Autodesk Inventor part; units mm, degrees
ref_plane "YZ Plane" through (0, 0, 0) normal (1, 0, 0) x (0, 1, 0)
ref_plane "XZ Plane" through (0, 0, 0) normal (0, 1, 0) x (-1, 0, 0)
ref_plane "XY Plane" through (0, 0, 0) normal (0, 0, 1) x (1, 0, 0)
sketch "Sketch3" plane through (0, 0, 0) normal (0, 0, 1) x (1, 0, 0)
  circle A0 centre (0, 0) radius 9.525
  dimension "d7" = 19.05
extrude "Extrusion3" add sketch "Sketch3" along normal blind 38.1
sketch "Sketch4" plane through (0, 0, 38.1) normal (0, 0, 1) x (1, 0, 0)
  line L0 (5.2594, 3.6744) -> (5.8118, -2.7176)
  line L1 (5.8118, -2.7176) -> (0.5524, -6.392)
  line L2 (0.5524, -6.392) -> (-5.2594, -3.6744)
  line L3 (-5.2594, -3.6744) -> (-5.8118, 2.7176)
  line L4 (-5.8118, 2.7176) -> (-0.5524, 6.392)
  line L5 (-0.5524, 6.392) -> (5.2594, 3.6744)
  point P0 (0, 0)
  point P1 (0, 0)
  dimension "d10" = 11.1125
extrude "Extrusion4" cut sketch "Sketch4" against normal blind 5.715
sketch "Sketch5" plane through (0, 0, 32.385) normal (0, 0, 1) x (1, 0, 0)
  circle A0 centre (0, 0) radius 2.3749
  dimension "d13" = 4.7498
hole "Hole1" at (0, 0, 32.385) direction (0, 0, -1) diameter 4.7498 depth 13.335 tip angle 118
sketch "Sketch6" plane through (0, 0, 0) normal (0, 0, -1) x (-1, 0, 0)
  point P0 (0, 0)
sketch "Sketch7" plane through (0, 0, 0) normal (0, 0, -1) x (-1, 0, 0)
  point P0 (0, 0)
sketch "Sketch8" plane through (0, 0, 0) normal (0, 0, -1) x (-1, 0, 0)
  arc A0 (-1.6801, 1.905) -> (1.6801, 1.905) centre (0, 0) ccw
  line L0 (-1.6801, 1.905) -> (1.6801, 1.905)
  dimension "d21" = 5.08
extrude "Extrusion5" cut sketch "Sketch8" against normal blind 19.05
properties part number "Vertical Sedder motor and rail coupler"
Design review of the part built by this model. Coordinates are the model's own, in mm. A direction names the side the tool comes from. Coordinates: 2 decimals unless noted, no trailing zeros. Order: outer loops, then holes, each group sorted by start corner. A loop starts at its lowest first (then second) coordinate and runs counter-clockwise, first axis right, second up. Notation, with made-up numbers: M 24.25,-38 L 83.25,-38 A10 ccw 83.25,-21 Z; hole C 50.25,86.5 d8. An arc over 180 degrees is marked long. Answer as a JSON object with one key per item and string values. Group by question number.
1) Add section A-A, the plane z = 34. Write out the cut boundary in (x, y) (3 decimals), then the cut area to 3 significant figures.
2) Wall thickness on L1, parallel to Y at x = 0, z = 14.25 (3 decimals); L2, parallel to Y at x = 0, z = 22.5 (3 decimals); L3, parallel to Z at x = -2.75, y = -3.5 (3 decimals): over which ranges is each line inside the solid? List them lowest first.
3) Add section D-D, the plane x = 3.5. Write out the cut boundary in (y, z) (3 decimals).
4) For pin 1 (8 mm diameter, centred on y = 7, z = 25, fed in from +X); pin 2 (6 mm diameter, centred on x = -4, z = 9.5, fed in from +Y); pin 3 (1.5 mm diameter, centred on y = -6, z = 12, fed in from -X), all flat-tipped, find the tip position at first contact; note any pin that passes through.
5) Add section B-B, the plane y = -1. Write out the cut boundary in (x, z) (3 decimals), then the cut area to 3 significant figures.
6) Mouldability with a two-part tool opening along X and no side actions: class faces 4 (the cylindrical face through (-7.559, 5.796, 18.783)), 5 (the flat face through (4.1, -4.1, 38.1)), 6 (the flat face through (-5.53, -0.52, 35.28)) as pulls with the +X half, pulls with the -X half, needs draft (parallel to the pull), parting line crosses it, or undercut.
7) Add section C-C, the plane x = 0. Write out the cut boundary in (y, z) (3 decimals), then the cut area to 3 significant figures.
8) Tool access review of faces 1 (the flat face through (-0.1, 2.3, 0)), 2 (the flat face through (0, 1.905, 9)), 3 (the flat face through (-2.313, -5.052, 35.283)): name each direction out of +Z, -Z, +X, -X, +Y, -Y from which nothing blocks a thin tool from reaching the whole face with its end or side.
Computed values:
{
 "1": {"outline": "C 0,0 d19.05; hole M -5.812,2.718 L -5.259,-3.674 L 0.552,-6.392 L 5.812,-2.718 L 5.259,3.674 L -0.552,6.392 Z", "area": "178 mm^2"},
 "2": {"L1": "y = -9.525 to -2.54, 1.905 to 9.525", "L2": "y = -9.525 to -2.375, 2.375 to 9.525", "L3": "z = 0 to 32.385"},
 "3": {"outline": "M -8.859,0 L 8.859,0 L 8.859,38.1 L 4.497,38.1 L 4.497,32.385 L -4.333,32.385 L -4.333,38.1 L -8.859,38.1 Z"},
 "4": {"pin 1": "stops at x = 9.04", "pin 2": "stops at y = 9.47", "pin 3": "stops at x = -7.95"},
 "5": {"outline": "M -9.472,0 L -2.335,0 L -2.335,19.05 L -2.154,19.05 L -2.154,32.385 L -5.491,32.385 L -5.491,38.1 L -9.472,38.1 Z; M 2.154,19.05 L 2.335,19.05 L 2.335,0 L 9.472,0 L 9.472,38.1 L 5.663,38.1 L 5.663,32.385 L 2.154,32.385 Z", "area": "512 mm^2"},
 "6": {"face 4": "parting line crosses it", "face 5": "needs draft", "face 6": "undercut"},
 "7": {"outline": "M -9.525,0 L -2.54,0 L -2.54,19.05 L -2.375,19.05 L -2.375,32.385 L -6.134,32.385 L -6.134,38.1 L -9.525,38.1 Z; M 1.905,0 L 9.525,0 L 9.525,38.1 L 6.134,38.1 L 6.134,32.385 L 2.375,32.385 L 2.375,19.05 L 1.905,18.768 Z", "area": "508 mm^2"},
 "8": {"face 1": "-Z, +X, -X, +Y, -Y", "face 2": "-Z", "face 3": "+Z"}
}
